from build123d import *

# Parameters (mm, degrees)
F0_W           = 15
F0_H           = 46
F0_R           = 2.5
F1_DEPTH       = 7
F2_DEPTH       = 19
F4_D           = 5.5
F4_CBORE_D     = 9.75
F4_CBORE_DEPTH = 5
F5_W           = 3
F5_H           = 8.2
F6_DEPTH       = 20
F8_D           = 6.6
F8_DEPTH       = 40
F8_CSINK_D     = 13.44
F8_CSINK_ANGLE = 90
F8_TIP         = 1.9828400428
F9_W           = 4.5
F9_H           = 3.8
F10_DEPTH      = 10


# Not quite as in the source:
# - a feature names something its author has since deleted; it is built from what else it names


with BuildPart() as f1:
    # F0 (on Top) → F1 (new body)
    with BuildSketch(Plane.XY):
        Polygon((-80, -60), (-80, 60), (-118, 60), (-118, 23), (-103, 23), (-103, -23), (-118, -23), (-118, -60), align=None)
        with BuildLine():
            Line((-86, -44.25), (-112, -44.25))
            ThreePointArc((-112, -44.25), (-117.25, -39), (-112, -33.75))
            Line((-112, -33.75), (-86, -33.75))
            ThreePointArc((-86, -33.75), (-80.75, -39), (-86, -44.25))
        make_face(mode=Mode.SUBTRACT)
        with BuildLine():
            Line((-86, 33.75), (-112, 33.75))
            ThreePointArc((-112, 33.75), (-117.25, 39), (-112, 44.25))
            Line((-112, 44.25), (-86, 44.25))
            ThreePointArc((-86, 44.25), (-80.75, 39), (-86, 33.75))
        make_face(mode=Mode.SUBTRACT)
        with Locations((-110.5, 0)):
            Rectangle(F0_W, F0_H)
        with BuildLine():
            ThreePointArc((-112, 44.25), (-117.25, 39), (-112, 33.75))
            Line((-112, 33.75), (-86, 33.75))
            ThreePointArc((-86, 33.75), (-80.75, 39), (-86, 44.25))
            Line((-86, 44.25), (-112, 44.25))
        make_face()
        with Locations((-112, 39)):
            Circle(F0_R, mode=Mode.SUBTRACT)
        with Locations((-86, 39)):
            Circle(F0_R, mode=Mode.SUBTRACT)
        with BuildLine():
            ThreePointArc((-112, -33.75), (-117.25, -39), (-112, -44.25))
            Line((-112, -44.25), (-86, -44.25))
            ThreePointArc((-86, -44.25), (-80.75, -39), (-86, -33.75))
            Line((-86, -33.75), (-112, -33.75))
        make_face()
        with Locations((-112, -39)):
            Circle(F0_R, mode=Mode.SUBTRACT)
        with BuildLine():
            ThreePointArc((-83.5, -39), (-86, -41.5), (-88.5, -39))
            ThreePointArc((-88.5, -39), (-86, -36.5), (-83.5, -39))
        make_face(mode=Mode.SUBTRACT)
        with Locations((-112, 39)):
            Circle(F0_R)
        with Locations((-86, 39)):
            Circle(F0_R)
        with Locations((-112, -39)):
            Circle(F0_R)
        with BuildLine():
            ThreePointArc((-83.5, -39), (-86, -36.5), (-88.5, -39))
            ThreePointArc((-88.5, -39), (-86, -41.5), (-83.5, -39))
        make_face()
    extrude(amount=-F1_DEPTH)

    # F0 (on Top) → F2 (join)
    with BuildSketch(Plane.XY):
        with BuildLine():
            ThreePointArc((-112, 44.25), (-117.25, 39), (-112, 33.75))
            Line((-112, 33.75), (-86, 33.75))
            ThreePointArc((-86, 33.75), (-80.75, 39), (-86, 44.25))
            Line((-86, 44.25), (-112, 44.25))
        make_face()
        with Locations((-112, 39)):
            Circle(F0_R, mode=Mode.SUBTRACT)
        with Locations((-86, 39)):
            Circle(F0_R, mode=Mode.SUBTRACT)
        with BuildLine():
            ThreePointArc((-112, -33.75), (-117.25, -39), (-112, -44.25))
            Line((-112, -44.25), (-86, -44.25))
            ThreePointArc((-86, -44.25), (-80.75, -39), (-86, -33.75))
            Line((-86, -33.75), (-112, -33.75))
        make_face()
        with Locations((-112, -39)):
            Circle(F0_R, mode=Mode.SUBTRACT)
        with BuildLine():
            ThreePointArc((-83.5, -39), (-86, -41.5), (-88.5, -39))
            ThreePointArc((-88.5, -39), (-86, -36.5), (-83.5, -39))
        make_face(mode=Mode.SUBTRACT)
        with Locations((-110.5, 0)):
            Rectangle(F0_W, F0_H)
        with Locations((-112, 39)):
            Circle(F0_R)
        with Locations((-86, 39)):
            Circle(F0_R)
        with BuildLine():
            ThreePointArc((-83.5, -39), (-86, -36.5), (-88.5, -39))
            ThreePointArc((-88.5, -39), (-86, -41.5), (-83.5, -39))
        make_face()
        with Locations((-112, -39)):
            Circle(F0_R)
    extrude(amount=F2_DEPTH)

    # F4 (through all)
    with Locations(Plane(origin=(-118, 0, 0), x_dir=(0, -1, 0), z_dir=(-1, 0, 0))):
        with Locations((-13, 9), (13, 9)):
            CounterBoreHole(F4_D / 2, F4_CBORE_D / 2, F4_CBORE_DEPTH)

    # F5 (on face) → F6 (cut)
    with BuildSketch(Plane.XY.offset(19)):
        with Locations((-109, 13)):
            Rectangle(F5_W, F5_H)
        with Locations((-109, -13)):
            Rectangle(F5_W, F5_H)
    extrude(amount=-F6_DEPTH, mode=Mode.SUBTRACT)

    # F8
    with Locations(Plane(origin=(0, 0, -7), x_dir=(1, 0, 0), z_dir=(0, 0, -1))):
        with Locations((-86, -39), (-112, -39), (-112, 39), (-86, 39)):
            CounterSinkHole(F8_D / 2, F8_CSINK_D / 2, depth=F8_DEPTH, counter_sink_angle=F8_CSINK_ANGLE)
            with Locations((0, 0, -(F8_DEPTH + F8_TIP / 2))):  # 118° drill point
                Cone(0, F8_D / 2, F8_TIP, mode=Mode.SUBTRACT)

    # F9 (on face) → F10 (cut)
    with BuildSketch(Plane.XY.offset(19)):
        with Locations((-105.25, 13)):
            Rectangle(F9_W, F9_H)
        with Locations((-105.25, -13)):
            Rectangle(F9_W, F9_H)
    extrude(amount=-F10_DEPTH, mode=Mode.SUBTRACT)


solid = f1.part
Design review of the part built by this model. Coordinates are the model's own, in mm. A direction names the side the tool comes from. Round coordinates to 2 decimals unless told otherwise and drop trailing zeros. Write each loop counter-clockwise with the first axis right and the second up, starting at its lowest first coordinate (ties: lowest second). Pieces come first, ordered by that corner, then holes.
Item 1: Draft analysis for pull direction Z (two halves, no side actions). For faces 5 (the cylindrical face through (-80.75, 38.88, 9.37)), 6 (the flat face through (-113, 10.9, 6.9)), 7 (the flat face through (-109, 13, -1)), state which applies: released by +Z, released by -Z, zero draft, split by the parting line, or undercut.
Item 2: For pin 1 Ø1 at (x, z) = (-86.5, 15.5) entering from -Y; pin 2 Ø5.5 at (x, y) = (-112, 39) entering from +Z; pin 3 Ø4 at (y, z) = (-36, 2.5) entering from -X; pin 4 Ø5 at (x, z) = (-104.5, 13.5) entering from +Y, all flat-tipped, find the tip position at first contact; note any pin that passes through.
Item 3: Consider section D-D on z = -2.25. Give the boundary of the cut face in (x, y).
Item 4: Consider section B-B on y = 13. Give the boundary of the cut face in (x, z) (3 decimals).
Item 5: Wall thickness on L1, parallel to Y at x = -86, z = 14; L2, parallel to Y at x = -112, z = 3.5; L3, parallel to Y at x = -108, z = 5.75: over which ranges is each line inside the solid? List them lowest first.
Item 6: Consider section C-C on y = 39. Give the boundary of the cut face in (x, z), and give its area (3 significant figures).
Item 7: For faces 1 (the cylindrical face through (-117.25, -38.88, 9.37)), 2 (the cylindrical face through (-115.54, 14.06, 4.24)), 3 (the flat face through (-109, 17.1, 9)), 4 (the cylindrical face through (-80.75, -39.12, 9.37)), list the 3-axis set-ups (+Z, -Z, +X, -X, +Y, -Y) from which the entire face can be reached by the end or side of a thin tool; tool diameter is ignored.
Item 8: Consider section A-A on z = 16.25. Count the separate pieces of the cut face and the enclosed holes in it, and give its area (3 significant figures).
Check values:
1. face 5: zero draft
1. face 6: undercut
1. face 7: released by +Z
2. pin 1: stops at y = -44.25
2. pin 2: passes through
2. pin 3: stops at x = -117.15
2. pin 4: stops at y = 44.25
3. outline: (-118, -60) - (-80, -60) - (-80, 60) - (-118, 60) - close; hole circle Ø6.6 at (-112, -39); hole circle Ø6.6 at (-112, 39); hole circle Ø6.6 at (-86, -39); hole circle Ø6.6 at (-86, 39)
4. outline: (-118, -7) - (-80, -7) - (-80, 0) - (-103, 0) - (-103, 6.25) - (-107.5, 6.25) - (-107.5, -1) - (-110.5, -1) - (-110.5, 6.25) - (-113, 6.25) - (-113, 4.125) - (-118, 4.125) - close; (-118, 13.875) - (-113, 13.875) - (-113, 11.75) - (-110.5, 11.75) - (-110.5, 19) - (-118, 19) - close
5. L1: y = -44.25 to -42.3, -35.7 to -33.75, 33.75 to 35.7, 42.3 to 44.25
5. L2: y = -44.25 to -42.3, -35.7 to -33.75, -23 to 23, 33.75 to 35.7, 42.3 to 44.25
5. L3: y = -44.25 to -33.75, -23 to -17.1, -8.9 to 8.9, 17.1 to 23, 33.75 to 44.25
6. outline: (-118, -6.28) - (-115.3, -3.58) - (-115.3, 19) - (-117.25, 19) - (-117.25, 0) - (-118, 0) - close; (-108.7, -3.58) - (-105.28, -7) - (-92.72, -7) - (-89.3, -3.58) - (-89.3, 19) - (-108.7, 19) - close; (-82.7, -3.58) - (-80, -6.28) - (-80, 0) - (-80.75, 0) - (-80.75, 19) - (-82.7, 19) - close
6. area: 593 mm2
7. face 1: +Z, -X
7. face 2: -X
7. face 3: +Z
7. face 4: +Z, +X
8. separate pieces: 3
8. enclosed holes: 4
8. area: 1,190 mm2
